The listing builds one solid part. Answer for the finished solid, in the listing's coordinates (mm). A direction names the side the tool comes from. Round coordinates to 2 decimals unless told otherwise and drop trailing zeros. Order: outer loops, then holes, each group sorted by start corner. A loop starts at its lowest first (then second) coordinate and runs counter-clockwise, first axis right, second up. Notation, with made-up numbers: (13, 21.25) - (38, 21.25) arc R19 cw to (38, 45.25) - close; hole circle Ø4 at (61, 16.5). An arc over 180 degrees is marked (long way). One line per item, written item: value. Start each with the question number.
1. For a pull along Z with two mould halves and no side action, classify faces 1 (the flat face through (54.286, 33.718, 2.296)), 2 (the cylindrical face through (55.77, -64.15, -55.02)), 3 (the flat face through (0, 3, -57)) as released by +Z, released by -Z, zero draft, split by the parting line, or undercut.
2. Section B-B, the plane y = 27 is taken. Give the vertices of the cut face in (x, z).
3. A tool of negligible diameter and unlimited length cuts with its end or side. For faces 4 (the flat face through (54.286, 13.267, -98.187)), 5 (the flat face through (54.29, 49.01, -79.84)), 6 (the flat face through (55, 68.784, 11)), 7 (the cylindrical face through (2.028, -8.675, -113.503)), 8 (the cylindrical face through (34.06, -64.42, -93.24)), from which of +Z, -Z, +X, -X, +Y, -Y can it reach the whole face along a straight path? Write none if from no direction.
4. Flat-ended cylindrical pins translate along their axes: P1, Ø6, axis at x = 66.5, y = -41.5, coming from the +Z side; P2, Ø1.8, axis at x = 60, z = -120.5, coming from the -Y side; P3, Ø10, axis at x = 59.5, z = -54, coming from the +Y side. Find the tip coordinate at first contact, or state that the pin passes through.
5. Section A-A, the plane z = -66 is taken. Give the vertices of the cut face in (x, y).
6. Straight lines are drawn through the part: line 1 (X direction, y = -20, z = -32); line 2 (Y direction, x = 60.5, z = -97); line 3 (Y direction, x = 19, z = -69). For each, find the intervals that lie inside material, in ascending order.
7. Section D-D, the plane y = -41 is taken. Give the vertices of the cut face in (x, z).
8. Section C-C, the plane x = 55 is taken. Count the separate pieces of the cut face and the enclosed holes in it, then the cut area to 3 significant figures.
from build123d import *

# Parameters (mm, degrees)
BOSS_EXTRUDE2_DEPTH = 110
CUT_EXTRUDE1_DEPTH  = 102
CUT_EXTRUDE2_START  = -60
CUT_EXTRUDE2_DEPTH  = 60
FILLET1_R           = 10
SKETCH9_R           = 2.15
CUT_EXTRUDE3_DEPTH  = 4
SKETCH10_R          = 2.15
CUT_EXTRUDE4_DEPTH  = 4
CHAMFER1_SIZE       = 2.6
SKETCH12_R          = 2.15
CUT_EXTRUDE5_DEPTH  = 180.904594821


with BuildPart() as part:
    # Sketch3 → Boss-Extrude2 (new body)
    with BuildSketch(Plane(origin=(0, 0, 0), x_dir=(0, 0, -1), z_dir=(1, 0, 0))):
        Polygon((-12.988659511, 68.784407565), (89.636946823, 68.784407565), (80, 34.980398699), (124.636946823, -5.113777665), (124.636946823, -65.113777665), (54.636946823, -65.113777665), (0, 0), align=None)
    extrude(amount=BOSS_EXTRUDE2_DEPTH)

    # Sketch5 → Cut-Extrude1 (cut)
    with BuildSketch(Plane.ZY.offset(-4)):
        Polygon((-84.337245247, 64.784407565), (-84.337245247, 68.784407565), (8.162643706, 68.784407565), (8.162643706, 64.784407565), (-3.736468645, 1.769945376), (-56.502177456, -61.113777665), (-120.636946823, -61.113777665), (-124.636946823, -61.113777665), (-124.636946823, -10.490489494), (-75.468261848, 33.674223088), align=None)
    extrude(amount=-CUT_EXTRUDE1_DEPTH, mode=Mode.SUBTRACT)

    # Sketch8 → Cut-Extrude2 (cut)
    with BuildSketch(Plane.XZ.offset(65.113777665).offset(CUT_EXTRUDE2_START)):
        with BuildLine():
            Line((0, -124.636946823), (110, -124.636946823))
            ThreePointArc((110, -124.636946823), (55, -99.101987445), (0, -124.636946823))
        make_face()
    extrude(amount=CUT_EXTRUDE2_DEPTH, mode=Mode.SUBTRACT)

    # Fillet1
    fillet1_edges = [part.edges().sort_by_distance(p)[0] for p in [
        (55, 34.980398699, -80),
        (55, -65.113777665, -54.636946823),
        (55, 0, 0),
    ]]
    fillet(fillet1_edges, radius=FILLET1_R)

    # Sketch9 → Cut-Extrude3 (cut)
    with BuildSketch(Plane.XZ.offset(65.113777665)):
        with Locations(Location((55, -91.601987445, 0), (0, 0, 270))):
            Circle(SKETCH9_R)
        with Locations(Location((77.397738269, -94.822296043, 0), (0, 0, 270))):
            Circle(SKETCH9_R)
        with Locations(Location((97.980944988, -104.222331585, 0), (0, 0, 270))):
            Circle(SKETCH9_R)
        with Locations((-23.69080463, -159.787957803)):
            Circle(SKETCH9_R)
        with Locations((-17.315743631, -138.076493912)):
            Circle(SKETCH9_R)
        with Locations((-5.082091161, -119.040559097)):
            Circle(SKETCH9_R)
        with Locations(Location((12.019055012, -104.222331585, 0), (0, 0, 270))):
            Circle(SKETCH9_R)
        with Locations(Location((32.602261731, -94.822296043, 0), (0, 0, 270))):
            Circle(SKETCH9_R)
    extrude(amount=-CUT_EXTRUDE3_DEPTH, mode=Mode.SUBTRACT)

    # Sketch10 → Cut-Extrude4 (cut)
    with BuildSketch(Plane(origin=(0, 59.13096402, -53.113115226), x_dir=(1, 0, 0), z_dir=(0, 0.7439491137225913, -0.6682362727294672))):
        with Locations(Location((55, 88.140757853, 0), (0, 0, 270))):
            Circle(SKETCH10_R)
        with Locations(Location((75, 88.140757853, 0), (0, 0, 270))):
            Circle(SKETCH10_R)
        with Locations(Location((95, 88.140757853, 0), (0, 0, 270))):
            Circle(SKETCH10_R)
        with Locations(Location((35, 88.140757853, 0), (0, 0, 270))):
            Circle(SKETCH10_R)
        with Locations(Location((15, 88.140757853, 0), (0, 0, 270))):
            Circle(SKETCH10_R)
    extrude(amount=-CUT_EXTRUDE4_DEPTH, mode=Mode.SUBTRACT)

    # Chamfer1
    chamfer1_edges = [part.edges().sort_by_distance(p)[0] for p in [
        (97.980944988, -61.113777665, -102.072331585),
        (77.397738269, -61.113777665, -92.672296043),
        (12.019055012, -61.113777665, -102.072331585),
        (32.602261731, -61.113777665, -92.672296043),
        (55, -61.113777665, -89.451987445),
    ]]
    chamfer(chamfer1_edges, length=CHAMFER1_SIZE)

    # Sketch12 → Cut-Extrude5 (cut, through all)
    with BuildSketch(Plane(origin=(110, 0, 0), x_dir=(0, 0, -1), z_dir=(1, 0, 0))):
        with Locations((113.968990901, -26.575845979)):
            Circle(SKETCH12_R)
        with Locations((113.968990901, -6.575845979)):
            Circle(SKETCH12_R)
        with Locations((113.968990901, -46.575845979)):
            Circle(SKETCH12_R)
    extrude(amount=-CUT_EXTRUDE5_DEPTH, mode=Mode.SUBTRACT)


solid = part.part
Answer list:
1. face 1: undercut
1. face 2: released by +Z
1. face 3: zero draft
2. outline: (0, -88.88) - (110, -88.88) - (110, 5.1) - (0, 5.1) - close; hole (4, -82.9) - (106, -82.9) - (106, 1.03) - (4, 1.03) - close
3. face 4: none
3. face 5: +Y
3. face 6: +Z, -Z, +X, -X, +Y
3. face 7: +X, -X
3. face 8: -Y
4. P1: stops at z = -32.31
4. P2: stops at y = -5.11
4. P3: stops at y = -52.17
5. outline: (0, -65.11) - (110, -65.11) - (110, 68.78) - (106, 68.78) - (106, -61.11) - (4, -61.11) - (4, 68.78) - (0, 68.78) - close
6. line 1: x = 0 to 4, 106 to 110
6. line 2: y = -65.11 to -61.11, 14.33 to 19.71
6. line 3: y = -65.11 to -61.11
7. outline: (0, -124.64) arc R72 cw to (4, -120.28) - (4, -39.62) - (106, -39.62) - (106, -120.28) arc R72 cw to (110, -124.64) - (110, -34.4) - (0, -34.4) - close
8. separate pieces: 4
8. enclosed holes: 0
8. area: 1,130 mm²
